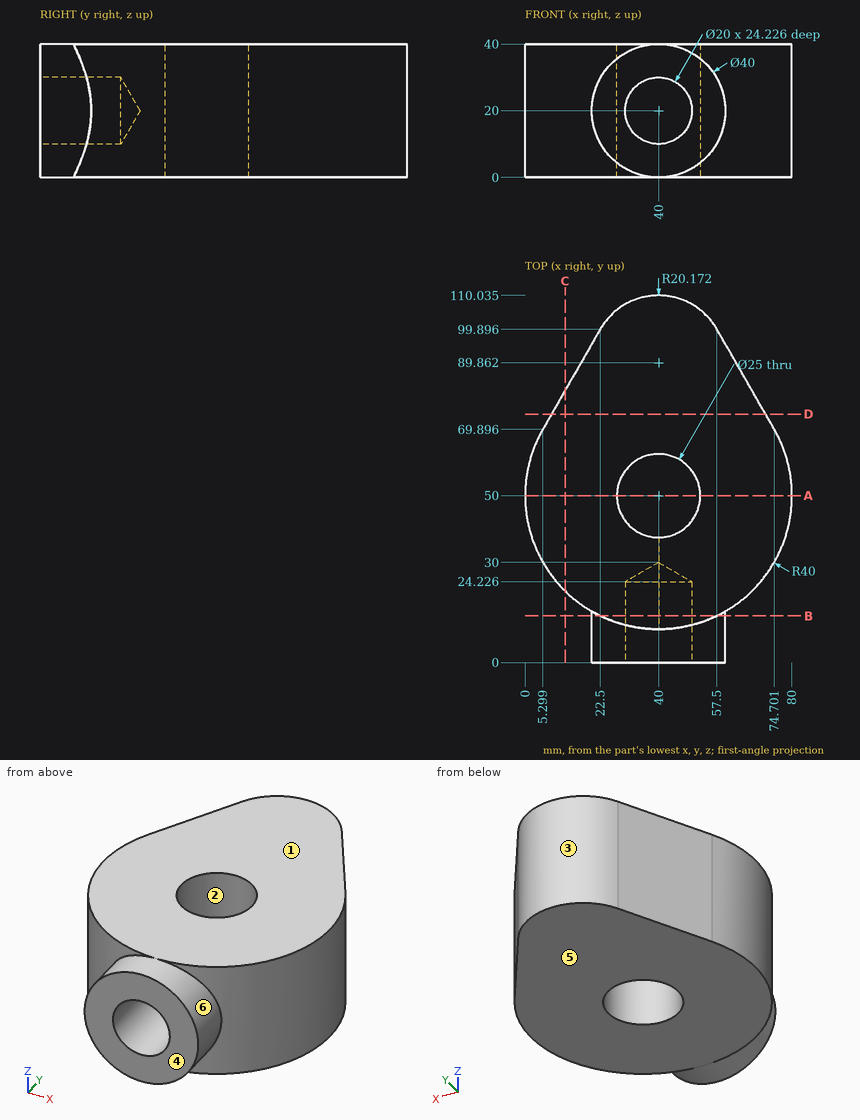
Design review of the part shown in the three views and the two pictorial views. Dimensions are in mm from the part's minimum x, y and z. A direction names the side the tool comes from. Round coordinates to 2 decimals unless told otherwise and drop trailing zeros. Loops run counter-clockwise (first coordinate to the right, second up) from the corner with the lowest first, then second, coordinate; pieces in that order, holes last. Notation, with made-up numbers: (30.5, -9.5) - (72.5, -9.5) arc R14 cw to (72.5, 10.5) - close; hole circle Ø7 at (-33, 86). An arc over 180 degrees is marked (long way). Write each question's results on one line, items separated by ' | '. Start each with the question number.
Q1. Insertion check: P1, Ø10, axis at x = 14.5, z = 4.5, coming from the -Y side; P2, Ø5, axis at y = 62.5, z = 33.5, coming from the +X side; P3, Ø6, axis at y = 29, z = 4.5, coming from the -X side; P4, Ø23, axis at x = 40, z = 20, coming from the -Y side. Each pin has a flat end and moves straight along its axis. Give the tip position at first contact, or say it passes through.
Q2. Take a section at D-D on y = 74.5. Give the boundary of the cut face in (x, z), plus the area to 4 significant figures.
Q3. Draft analysis for pull direction Y (two halves, no side actions). For the marked faces 1, 2, 3 and 4, state which applies: pulls with the +Y half, pulls with the -Y half, needs draft (parallel to the pull), parting line crosses it, or undercut.
Q4. Take a section at C-C on x = 12. Give the boundary of the cut face in (y, z) (1 decimal), plus the area to 3 significant figures.
Q5. Take a section at A-A on y = 50. Give the boundary of the cut face in (x, z), plus the area to 3 significant figures.
Q6. Wall thickness on line 1 along X through (y, z) = (10, 20); line 2 along X through (y, z) = (54.5, 34.5) (1 decimal); line 3 along Y through (x, z) = (31, 8.5) (1 decimal): over which ranges is each line inside the solid? List them lowest first. Write a range as [from, to].
Q7. Tool access review of the marked faces 5 and 6: name each direction out of +Z, -Z, +X, -X, +Y, -Y from which nothing blocks a thin tool from reaching the whole face with its end or side.
Q8. Take a section at B-B on y = 14. Give the boundary of the cut face in (x, z) (1 decimal).
Data:
1) P1: stops at y = 15.65 | P2: stops at x = 78.73 | P3: stops at x = 4.28 | P4: stops at y = 0
2) outline: (7.94, 0) - (72.06, 0) - (72.06, 40) - (7.94, 40) - close | area: 2,565 mm²
3) face 1: needs draft | face 2: undercut | face 3: pulls with the +Y half | face 4: pulls with the -Y half
4) outline: (21.4, 0) - (81.6, 0) - (81.6, 40) - (21.4, 40) - close | area: 2,410 mm²
5) outline: (0, 0) - (27.5, 0) - (27.5, 40) - (0, 40) - close; (52.5, 0) - (80, 0) - (80, 40) - (52.5, 40) - close | area: 2,200 mm²
6) line 1: x = [20, 30], [50, 60] | line 2: x = [0.3, 28.3], [51.7, 79.7] | line 3: y = [0, 41.3], [58.7, 107.9]
7) face 5: -Z, +X, -X, +Y, -Y | face 6: -Y
8) outline: (22.6, 0) - (57.4, 0) - (57.4, 10.2) arc R20 ccw to (57.4, 29.8) - (57.4, 40) - (22.6, 40) - (22.6, 29.8) arc R20 ccw to (22.6, 10.2) - close; hole circle Ø20 at (40, 20)
